```python
from build123d import *

# Parameters (mm, degrees)
SKETCH1_W           = 400
SKETCH1_H           = 200
SKETCH1_W_2         = 390
SKETCH1_H_2         = 190
BOSS_EXTRUDE1_DEPTH = 300
CUT_EXTRUDE1_REACH  = 414.311
SKETCH7_R           = 63.5
SKETCH8_W           = 400
SKETCH8_H           = 200
BOSS_EXTRUDE2_DEPTH = 0.5


with BuildPart() as part:
    # Sketch1 → Boss-Extrude1 (new body)
    with BuildSketch(Plane(origin=(0, 0, 0), x_dir=(1, 0, 0), z_dir=(0, 1, 0))):
        Rectangle(SKETCH1_W, SKETCH1_H)
        Rectangle(SKETCH1_W_2, SKETCH1_H_2, mode=Mode.SUBTRACT)
    extrude(amount=BOSS_EXTRUDE1_DEPTH)

    # Sketch7 → Cut-Extrude1 (cut, up to next)
    with BuildSketch(Plane.XY.offset(100), mode=Mode.PRIVATE) as cut_extrude1_sk1:
        with Locations((-123.8, 223.8)):
            Circle(SKETCH7_R)
    cut_extrude1_tool1 = extrude(cut_extrude1_sk1.sketch, amount=-CUT_EXTRUDE1_REACH, mode=Mode.PRIVATE) & part.part
    add(cut_extrude1_tool1.solids().sort_by_distance((-123.8, 223.8, 100))[0], mode=Mode.SUBTRACT)

    # Sketch8 → Boss-Extrude2 (add)
    with BuildSketch(Plane.XZ):
        Rectangle(SKETCH8_W, SKETCH8_H)
    extrude(amount=-BOSS_EXTRUDE2_DEPTH)


solid = part.part
```
Work out the finished part from the listing and answer in its coordinate system (mm). A direction names the side the tool comes from. Give positions to 0.01 mm unless a question says otherwise; leave off trailing zeros. Order: outer loops, then holes, each group sorted by start corner. A loop starts at its lowest first (then second) coordinate and runs counter-clockwise, first axis right, second up.
1. Section C-C, the plane x = 61.5 is taken. Determine the outline of the cut face in (y, z).
Result sheet:
outline: (0, -100) - (300, -100) - (300, -95) - (0.5, -95) - (0.5, 95) - (300, 95) - (300, 100) - (0, 100) - close
2. Straight lines are drawn through the part: L1, parallel to Z at x = -133, y = 20; L2, parallel to X at y = 138, z = -71; L3, parallel to X at y = 223, z = 96. For each, find the intervals that lie inside material, in ascending order.
Result sheet:
L1: z = -100 to -95, 95 to 100
L2: x = -200 to -195, 195 to 200
L3: x = -200 to -187.29, -60.31 to 200
3. For faces 5 (the flat face through (-3, 148, 100)), 6 (the flat face through (-3, 0.5, 1)), 7 (the cylindrical face through (-137.57, 161.81, 97.54)), determine the directions among +Z, -Z, +X, -X, +Y, -Y from which every point of the face is accessible in a straight line to the end or side of a thin tool.
Result sheet:
face 5: +Z, +X, -X, +Y, -Y
face 6: +Y
face 7: +Z
4. Section B-B, the plane y = 223.8 is taken. Determine the outline of the cut face in (x, z).
Result sheet:
outline: (-200, -100) - (200, -100) - (200, 100) - (-60.3, 100) - (-60.3, 95) - (195, 95) - (195, -95) - (-195, -95) - (-195, 95) - (-187.3, 95) - (-187.3, 100) - (-200, 100) - close
5. This flat-tipped pin is pushed along its axis until it touches: P1, Ø2, axis at x = -140, y = 163.5, coming from the +Z side. Where does it stop, or does it pass through?
Result sheet:
P1: stops at z = -95
6. Section D-D, the plane y = 73.5 is taken. Determine the outline of the cut face in (x, z), and give its area (3 significant figures).
Result sheet:
outline: (-200, -100) - (200, -100) - (200, 100) - (-200, 100) - close; hole (-195, -95) - (195, -95) - (195, 95) - (-195, 95) - close
area: 5,900 mm2
7. Section A-A, the plane x = -123.8 is taken. Determine the outline of the cut face in (y, z).
Result sheet:
outline: (0, -100) - (300, -100) - (300, -95) - (0.5, -95) - (0.5, 95) - (160.3, 95) - (160.3, 100) - (0, 100) - close; (287.3, 95) - (300, 95) - (300, 100) - (287.3, 100) - close
8. The mould has two halves that part along X. Classify faces 1 (the flat face through (-3, 0, -1)), 2 (the flat face through (-200, 148, 1)), 3 (the flat face through (200, 148, 1)), 4 (the flat face through (-195, 148, 1)): released by +X, released by -X, zero draft, split by the parting line, or undercut.
Result sheet:
face 1: zero draft
face 2: released by -X
face 3: released by +X
face 4: undercut
